Design review of the part built by this model. Coordinates are the model's own, in mm. A direction names the side the tool comes from. Give positions to 0.01 mm unless a question says otherwise; leave off trailing zeros. Answer in a Markdown table with one row per item. Add a question column.
Autodesk Inventor part; units mm, degrees
ref_plane "YZ Plane" through (0, 0, 0) normal (1, 0, 0) x (0, 1, 0)
ref_plane "XZ Plane" through (0, 0, 0) normal (0, 1, 0) x (-1, 0, 0)
ref_plane "XY Plane" through (0, 0, 0) normal (0, 0, 1) x (1, 0, 0)
sketch "Sketch1" plane through (0, 0, 0) normal (0, 0, 1) x (1, 0, 0)
  line L0 (14.98, 33.7) -> (197.7852, 33.7)
  line L1 (197.7852, 8.3) -> (14.98, 8.3)
  line L2 (14.98, 8.3) -> (14.98, 33.7)
  arc A0 (30.1177, 21.5547) -> (28.8951, 18.8151) centre (27.68, 21) ccw construction
  line L3 (30.1177, 21.5547) -> (28.8951, 18.8151) construction
  line L4 (-3.175, 42) -> (-122.9515, 42)
  line L5 (137.6968, 28.62) -> (137.6968, 13.38)
  line L6 (137.6968, 13.38) -> (122.4568, 28.62)
  line L7 (122.4568, 28.62) -> (137.6968, 28.62)
  line L8 (130.5126, 13.38) -> (115.2726, 28.62)
  line L9 (115.2726, 28.62) -> (115.2726, 13.38)
  line L10 (115.2726, 13.38) -> (130.5126, 13.38)
  line L11 (112.7326, 10.7487) -> (112.7326, 41.4812) construction
  line L12 (87.7684, 28.62) -> (87.7684, 13.38)
  line L13 (87.7684, 13.38) -> (103.0084, 28.62)
  line L14 (103.0084, 28.62) -> (87.7684, 28.62)
  line L15 (94.9526, 13.38) -> (110.1926, 28.62)
  line L16 (110.1926, 28.62) -> (110.1926, 13.38)
  line L17 (110.1926, 13.38) -> (94.9526, 13.38)
  line L18 (85.2284, 8.9371) -> (85.2284, 32.7241) construction
  line L19 (32.76, 28.62) -> (32.76, 13.38)
  line L20 (32.76, 13.38) -> (48, 28.62)
  line L21 (48, 28.62) -> (32.76, 28.62)
  line L22 (39.9442, 13.38) -> (55.1842, 28.62)
  line L23 (55.1842, 28.62) -> (55.1842, 13.38)
  line L24 (55.1842, 13.38) -> (39.9442, 13.38)
  line L25 (82.6884, 28.62) -> (82.6884, 13.38)
  line L26 (82.6884, 13.38) -> (67.4484, 28.62)
  line L27 (67.4484, 28.62) -> (82.6884, 28.62)
  line L28 (75.5042, 13.38) -> (60.2642, 28.62)
  line L29 (60.2642, 13.38) -> (75.5042, 13.38)
  line L30 (60.2642, 28.62) -> (60.2642, 13.38)
  line L31 (140.2368, 33.7) -> (140.2368, 8.3) construction
  line L32 (142.7768, 28.62) -> (142.7768, 13.38)
  line L33 (142.7768, 13.38) -> (158.0168, 28.62)
  line L34 (158.0168, 28.62) -> (142.7768, 28.62)
  line L35 (149.961, 13.38) -> (165.201, 28.62)
  line L36 (165.201, 28.62) -> (165.201, 13.38)
  line L37 (165.201, 13.38) -> (149.961, 13.38)
  line L38 (192.7052, 28.62) -> (192.7052, 13.38)
  line L39 (192.7052, 13.38) -> (177.4652, 28.62)
  line L40 (177.4652, 28.62) -> (192.7052, 28.62)
  line L41 (185.521, 13.38) -> (170.281, 28.62)
  line L42 (170.281, 13.38) -> (185.521, 13.38)
  line L43 (170.281, 28.62) -> (170.281, 13.38)
  line L44 (197.7852, 33.7) -> (197.7852, 8.3)
  arc A1 (30.379, 21.5269) -> (29.0903, 18.6392) centre (27.68, 21) ccw
  line L45 (29.0903, 18.6392) -> (30.379, 21.5269)
  point P0 (0, 0)
  dimension "d0" = 12.7
  dimension "d1" = 12.7
  dimension "d2" = 12.7
  dimension "d7" = 45
  dimension "d9" = 5.08
  dimension "d10" = 5.08
  dimension "d11" = 5.08
  dimension "d12" = 0
  dimension "d14" = 2.54
  dimension "d15" = 2.54
  dimension "d16" = 5.08
  dimension "d23" = 2.54
  dimension "d24" = 5.08
  dimension "d29" = 5.5
  dimension "d30" = 2.5
  dimension "d31" = 0.25
extrude "Extrusion4" add sketch "Sketch1" along normal blind 6.35
fillet "Fillet7" radius 3.175 12 edges at (106.3826, 8.3, 6.35) (106.3826, 8.3, 0) (106.3826, 33.7, 0) (106.3826, 33.7, 6.35) (197.7852, 21, 6.35) (197.7852, 21, 0) (197.7852, 33.7, 3.175) (197.7852, 8.3, 3.175) (14.98, 21, 6.35) (14.98, 21, 0) (14.98, 8.3, 3.175) (14.98, 33.7, 3.175)
fillet "Fillet8" radius 3.175 12 edges at (55.1842, 13.38, 3.175) (60.2642, 13.38, 3.175) (32.76, 28.62, 3.175) (82.6884, 28.62, 3.175) (87.7684, 28.62, 3.175) (110.1926, 13.38, 3.175) (115.2726, 13.38, 3.175) (137.6968, 28.62, 3.175) (142.7768, 28.62, 3.175) (165.201, 13.38, 3.175) (170.281, 13.38, 3.175) (192.7052, 28.62, 3.175)
equation "\"d1\" = d0"
equation "\"d24\" = d9"
properties part number "endarm"
1) Mouldability with a two-part tool opening along X and no side actions: class faces 1 (the face through (15.89, 21.13, 5.4)), 2 (the face through (46, 13.38, 3)), 3 (the face through (105, 25, 0)) as +X half, -X half, draft (parallel to the pull), parting line (faces both ways), or undercut.
2) Add section C-C, the plane z = 4.25. Give the number of separate pieces and of enclosed holes in the cut face, and give its area (3 significant figures).
3) Machinability: for faces 4 (the face through (196.831, 20.867, 0.905)), 5 (the face through (130.183, 20.893, 3.131)), which of the approach directions +Z, -Z, +X, -X, +Y, -Y give a long, thin tool a straight path to every point of the face, cutting with its end or side? Answer none if there is none.
4) For L1, parallel to Y at x = 123.5, z = 5.75; L2, parallel to Y at x = 98, z = 3.25; L3, parallel to Y at x = 174, z = 3.25, list the stretches that pass through material, from the lowest coordinate up.
5) Clearance check with flat-ended pins moving along their axes: P1, Ø2, axis at y = 17, z = 5, coming from the -X side; P2, Ø2, axis at x = 83.5, z = 5.5, coming from the +Y side; P3, Ø1.9, axis at y = 20, z = 2, coming from the +X side. State where each tip first meets the part, or that it passes through.
Verdict:
| question | item | result |
|---|---|---|
| 1 | face 1 | -X half |
| 1 | face 2 | undercut |
| 1 | face 3 | draft |
| 2 | separate pieces | 1 |
| 2 | enclosed holes | 13 |
| 2 | area | 3,170 mm2 |
| 3 | face 4 | -Z, +X, +Y, -Y |
| 3 | face 5 | +Z, -Z |
| 4 | L1 | y = 9.62 to 13.38, 20.39 to 27.58, 28.62 to 32.38 |
| 4 | L2 | y = 8.3 to 13.38, 16.43 to 23.61, 28.62 to 33.7 |
| 4 | L3 | y = 8.3 to 13.38, 24.9 to 33.7 |
| 5 | P1 | stops at x = 15.09 |
| 5 | P2 | stops at y = 33.41 |
| 5 | P3 | stops at x = 197.78 |
